Could you check a few things on this model? Use its own coordinates, in mm. Face numbers are marked on the shaded views. Round coordinates to 2 decimals unless told otherwise and drop trailing zeros. Loops run counter-clockwise (first coordinate to the right, second up) from the corner with the lowest first, then second, coordinate; pieces in that order, holes last.
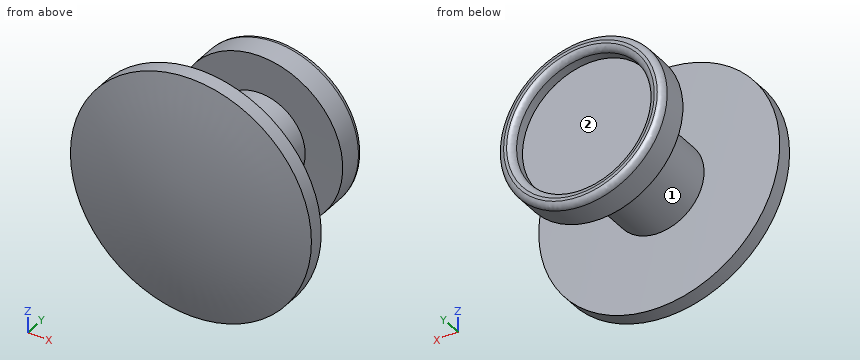
from build123d import *

# Parameters (mm, degrees)
CONG_1_R = 0.2


with BuildPart() as part:
    # Esquisse1 → Révolution1 (revolve)
    with BuildSketch(Plane.XY, mode=Mode.PRIVATE) as r_volution1_sk:
        with BuildLine():
            Line((-1.5, -1.002988992), (-1.5, -4.003013447))
            ThreePointArc((-1.5, -4.003013447), (-2.750015694, -4.010192747), (-4, -4.021595148))
            Line((-4, -4.021595148), (-4, -4.521595148))
            ThreePointArc((-4, -4.521595148), (-2.015564437, -4.896110644), (0, -5.021595148))
            Line((0, -5.021595148), (0, -0.50676811))
            Line((0, -0.50676811), (-2.25, -0.50676811))
            Line((-2.25, -0.50676811), (-2.25, -0.00676811))
            ThreePointArc((-2.25, -0.00676811), (-2.500000559, -0.008355713), (-2.75, -0.010110432))
            Line((-2.75, -0.010110432), (-2.75, -1.010110432))
            ThreePointArc((-2.75, -1.010110432), (-2.125002983, -1.006026077), (-1.5, -1.002988992))
        make_face()
    revolve(r_volution1_sk.sketch.rotate(Axis((0, 39.029541446, 0), (0, -1, 0)), 270), axis=Axis((0, 39.029541446, 0), (0, -1, 0)))  # turned: the seam where the file's is

    # Congé1
    cong_1_edges = [part.edges().sort_by_distance(p)[0] for p in [
        (0, -0.010110432, -2.75),
        (0, -0.00676811, -2.25),
    ]]
    fillet(cong_1_edges, radius=CONG_1_R)


solid = part.part
Item 1: Will these pins go through, and if not, where does the flat tip stop? pin 1 (1.5 mm diameter, centred on x = -3, z = -1, fed in from +Y); pin 2 (1 mm diameter, centred on x = -1.5, z = 0, fed in from -Y); pin 3 (1.5 mm diameter, centred on x = 1, y = -3.5, fed in from +Z).
Results list:
pin 1: stops at y = -0.01
pin 2: stops at y = -4.99
pin 3: stops at z = 3.97
Item 2: If I drill on line 1 along X through (y, z) = (-0.25, 0); line 2 along Y through (x, z) = (1.5, 1.5); line 3 along Y through (x, z) = (1.5, 2.25), over which ranges is the centre line in solid material (lowest first)?
Results list:
line 1: x = -2.75 to -2.25, 2.25 to 2.75
line 2: y = -4.88 to -4.01, -1.01 to -0.51
line 3: y = -4.8 to -4.01, -1.01 to -0.08
Item 3: If we section it at B-B, the plane y = -4.15: Please give me the cut outline in (x, z).
Results list:
outline: circle Ø8 at (0, 0)
Item 4: If we section it at A-A, the plane y = -1.6: Please give me the cut outline in (x, z), then the cut area to 3 significant figures.
Results list:
outline: circle Ø3 at (0, 0)
area: 7.07 mm2
Item 5: We'd pull the mould along Z, two halves only. Please class the marked faces 1 and 2: released by +Z, released by -Z, zero draft, split by the parting line, or undercut.
Results list:
face 1: split by the parting line
face 2: undercut
